from build123d import *

# Parameters (mm, degrees)
BASE_FLANGE1_DEPTH = 491.5
SKETCH3_W          = 127.454139471
SKETCH3_H          = 14.5
SKETCH3_W_2        = 136.466577612
CUT_EXTRUDE3_DEPTH = 500.481230879
CUT_EXTRUDE5_START = 421.5
CUT_EXTRUDE5_DEPTH = 65


# Read off the part's stored shape, not the designer's step: Cut-Extrude5
# Sheet-metal steps are written as plain solids
with BuildPart() as part:
    # Sketch1 → Base-Flange1 (new, symmetric)
    with BuildSketch(Plane(origin=(0, 0, 0), x_dir=(1, 0, 0), z_dir=(0, 1, 0))):
        with BuildLine():
            Line((9.5, 65), (9.5, 74.7634))
            ThreePointArc((9.5, 74.7634), (10.155084973, 76.344915027), (11.7366, 77))
            Line((11.7366, 77), (37.2634, 77))
            ThreePointArc((37.2634, 77), (38.844915027, 76.344915027), (39.5, 74.7634))
            Line((39.5, 74.7634), (39.5, 30))
            Line((39.5, 30), (39.5, 24))
            Line((39.5, 24), (39.5, 13.8))
            ThreePointArc((39.5, 13.8), (41.269678139, 12.091041686), (42.915834526, 13.91928357))
            Line((42.915834526, 13.91928357), (42.378230266, 21.607382671))
            ThreePointArc((42.378230266, 21.607382671), (42.973636332, 23.288757532), (44.609382021, 24))
            Line((44.609382021, 24), (51.7634, 24))
            ThreePointArc((51.7634, 24), (53.344915027, 23.344915027), (54, 21.7634))
            Line((54, 21.7634), (54, -30))
            Line((54, -30), (54, -74.7634))
            ThreePointArc((54, -74.7634), (53.344915027, -76.344915027), (51.7634, -77))
            Line((51.7634, -77), (39.5, -77))
            Line((39.5, -77), (11.7366, -77))
            ThreePointArc((11.7366, -77), (10.155084973, -76.344915027), (9.5, -74.7634))
            Line((9.5, -74.7634), (9.5, -65))
            Line((9.5, -65), (11, -65))
            Line((11, -65), (11, -74.7634))
            ThreePointArc((11, -74.7634), (11.215745145, -75.284254855), (11.7366, -75.5))
            Line((11.7366, -75.5), (39.5, -75.5))
            Line((39.5, -75.5), (51.7634, -75.5))
            ThreePointArc((51.7634, -75.5), (52.284254855, -75.284254855), (52.5, -74.7634))
            Line((52.5, -74.7634), (52.5, -30))
            Line((52.5, -30), (52.5, 21.7634))
            ThreePointArc((52.5, 21.7634), (52.284254855, 22.284254855), (51.7634, 22.5))
            Line((51.7634, 22.5), (44.609382021, 22.5))
            ThreePointArc((44.609382021, 22.5), (44.070666884, 22.265759992), (43.874576341, 21.712017381))
            Line((43.874576341, 21.712017381), (44.412180601, 14.023918281))
            ThreePointArc((44.412180601, 14.023918281), (41.322027384, 10.591955445), (38, 13.8))
            Line((38, 13.8), (38, 24))
            Line((38, 24), (38, 30))
            Line((38, 30), (38, 74.7634))
            ThreePointArc((38, 74.7634), (37.784254855, 75.284254855), (37.2634, 75.5))
            Line((37.2634, 75.5), (11.7366, 75.5))
            ThreePointArc((11.7366, 75.5), (11.215745145, 75.284254855), (11, 74.7634))
            Line((11, 74.7634), (11, 65))
            Line((11, 65), (9.5, 65))
        make_face()
    extrude(amount=BASE_FLANGE1_DEPTH, both=True)

    # Sketch3 → Cut-Extrude3 (cut, through all)
    with BuildSketch(Plane(origin=(54, 0, 0), x_dir=(0, 0, -1), z_dir=(1, 0, 0))):
        with Locations((-39.227069736, -484.25)):
            Rectangle(SKETCH3_W, SKETCH3_H)
        with Locations((-18.733288806, 484.25)):
            Rectangle(SKETCH3_W_2, SKETCH3_H)
    extrude(amount=-CUT_EXTRUDE3_DEPTH, mode=Mode.SUBTRACT)

    # Cut-Extrude5 outline → Cut-Extrude5 (cut)
    with BuildSketch(Plane(origin=(0, 0, 0), x_dir=(1, 0, 0), z_dir=(0, 1, 0)).offset(CUT_EXTRUDE5_START)):
        with BuildLine():
            Line((37.2634, 77), (24.859115026, 77))
            Line((24.859115026, 77), (24.859115026, 75.5))
            Line((24.859115026, 75.5), (37.2634, 75.5))
            ThreePointArc((37.2634, 75.5), (37.755935518, 75.311111898), (37.995866912, 74.841321649))
            Line((37.995866912, 74.841321649), (39.487450359, 75))
            ThreePointArc((39.487450359, 75), (38.758926663, 76.426463306), (37.2634, 77))
        make_face()
    extrude(amount=CUT_EXTRUDE5_DEPTH, mode=Mode.SUBTRACT)


solid = part.part
The listing builds one solid part. Answer for the finished solid, in the listing's coordinates (mm). A direction names the side the tool comes from. Give positions to 0.01 mm unless a question says otherwise; leave off trailing zeros. Order: outer loops, then holes, each group sorted by start corner. A loop starts at its lowest first (then second) coordinate and runs counter-clockwise, first axis right, second up. Notation, with made-up numbers: (68, 12.5) - (74, 12.5) arc R14 cw to (74, 21.5) - close; hole circle Ø8 at (1.25, 62.5). An arc over 180 degrees is marked (long way). One line per item, written item: value. Start each with the question number.
1) The mould has two halves that part along Z. Classify faces 6 (the face through (31, 7, 75.5)), 7 (the face through (39, -491.5, -64)), 8 (the face through (24, 7, -77)), 9 (the face through (38, 7, -44)): released by +Z, released by -Z, zero draft, split by the parting line, or undercut.
2) Find the intervals of material crossed by L1, parallel to Z at x = 32.5, y = 9; L2, parallel to Z at x = 51.5, y = 35.5; L3, parallel to X at y = -223, z = 68, in increasing order.
3) A cutting plane is placed at C-C on z = -36.5. Give the vertices of the cut face in (x, y).
4) A tool of negligible diameter and unlimited length cuts with its end or side. For faces 1 (the face through (54, 7, 26)), 2 (the face through (53, -477, 23)), 3 (the face through (25, 7, -75.5)), 4 (the face through (27, 491.5, -76)), 5 (the face through (53, 477, 9)), from which of +Z, -Z, +X, -X, +Y, -Y can it reach the whole face along a straight path? Write none if from no direction.
5) Given pin 1 Ø5.5 at (x, y) = (49, 93.5) entering from -Z; pin 2 Ø1.2 at (x, y) = (10.5, -110.5) entering from -Z; pin 3 Ø1.2 at (x, y) = (38.5, -485) entering from +Z, each flat-ended and moving along its own axis, determine where each tip first touches the part or whether it passes through.
6) A cutting plane is placed at B-B on z = 50. Give the vertices of the cut face in (x, y), then the cut area to 3 significant figures.
Answer sheet:
1. face 6: undercut
1. face 7: zero draft
1. face 8: released by -Z
1. face 9: undercut
2. L1: z = -77 to -75.5, 75.5 to 77
2. L2: z = -24 to -22.5, 75.5 to 77
2. L3: x = 9.5 to 11, 52.5 to 54
3. outline: (38, -491.5) - (39.5, -491.5) - (39.5, 477) - (38, 477) - close
4. face 1: +Z, -Z, +X, +Y, -Y
4. face 2: +Z, +X, -X, -Y
4. face 3: +Y, -Y
4. face 4: +Z, -Z, +X, -X, +Y
4. face 5: +Z, +X, -X, +Y
5. pin 1: stops at z = -24
5. pin 2: stops at z = -76.91
5. pin 3: stops at z = -24.5
6. outline: (52.5, -477) - (54, -477) - (54, 477) - (52.5, 477) - close
6. area: 1,430 mm2
